Source: CAD feature listing. Evaluate the final solid. Frame: model axes, mm. A direction names the side the tool comes from. Give positions to 0.01 mm unless a question says otherwise; leave off trailing zeros. Order: outer loops, then holes, each group sorted by start corner. A loop starts at its lowest first (then second) coordinate and runs counter-clockwise, first axis right, second up.
```python
from build123d import *

# Parameters (mm, degrees)
SKETCH1_R                = 2.65
SKETCH1_R_2              = 1.65
BOSS_EXTRUDE1_DEPTH      = 6
SKETCH2_W                = 3
SKETCH2_H                = 84
BOSS_EXTRUDE2_DEPTH      = 5
BOSS_EXTRUDE2_DEPTH_BACK = 11
SKETCH3_W                = 3.872725059
SKETCH3_H                = 4
CUT_EXTRUDE2_DEPTH       = 10
CUT_EXTRUDE2_DEPTH_BACK  = 20


with BuildPart() as part:
    # Sketch1 → Boss-Extrude1 (new body)
    with BuildSketch(Plane(origin=(0, 0, 0), x_dir=(1, 0, 0), z_dir=(0, 1, 0))):
        with BuildLine():
            Line((10, 0), (0, 0))
            Line((0, 0), (0, -84))
            add(Edge.make_bspline(
                [(10, 0), (21.928320777, -51.98362607), (0, -84)],
                knots=[0, 0, 0, 0.5770461, 0.5770461, 0.5770461], degree=2))
        make_face()
        with Locations((7.5, -42.64)):
            Circle(SKETCH1_R, mode=Mode.SUBTRACT)
        with Locations((7.5, -17.64)):
            Circle(SKETCH1_R_2, mode=Mode.SUBTRACT)
    extrude(amount=BOSS_EXTRUDE1_DEPTH)

    # Sketch2 → Boss-Extrude2 (add, two sides)
    with BuildSketch(Plane(origin=(0, 6, 0), x_dir=(1, 0, 0), z_dir=(0, 1, 0))) as boss_extrude2_sk:
        with Locations((-1.5, -42)):
            Rectangle(SKETCH2_W, SKETCH2_H)
    extrude(amount=BOSS_EXTRUDE2_DEPTH)
    extrude(boss_extrude2_sk.sketch, amount=-BOSS_EXTRUDE2_DEPTH_BACK)

    # Sketch3 → Cut-Extrude2 (cut, two sides)
    with BuildSketch(Plane(origin=(0, 6, 0), x_dir=(1, 0, 0), z_dir=(0, 1, 0))) as cut_extrude2_sk:
        Polygon((23.981174241, 0), (0, 0), (0, -4), (0, -10), (23.981174241, -10), align=None)
        with Locations((-1.93636253, -2)):
            Rectangle(SKETCH3_W, SKETCH3_H)
    extrude(amount=CUT_EXTRUDE2_DEPTH, mode=Mode.SUBTRACT)
    extrude(cut_extrude2_sk.sketch, amount=-CUT_EXTRUDE2_DEPTH_BACK, mode=Mode.SUBTRACT)


solid = part.part
```
1) Section query A-A, the plane y = 5. Count the separate pieces of the cut face and the enclosed holes in it, and give its area (3 significant figures).
Report:
separate pieces: 1
enclosed holes: 2
area: 1,030 mm2
2) Reachability of faces 4 (the flat face through (6, 3, 10)), 5 (the flat face through (5, 6, 38)), 6 (the flat face through (-2, 3, 84)), 7 (the flat face through (5, 0, 38)), 8 (the flat face through (-2, 11, 43)) from +Z, -Z, +X, -X, +Y, -Y: full face, straight path, thin tool, end or side. Return the list, or none.
Report:
face 4: -Z, +X, +Y, -Y
face 5: +Z, -Z, +X, +Y
face 6: +Z, +X, -X, +Y, -Y
face 7: +Z, -Z, +X, -Y
face 8: +Z, -Z, +X, -X, +Y
3) Draft query along X for faces 1 (the flat face through (-3, 3, 45)), 2 (the cylindrical face through (7.14, 2.96, 19.25)), 3 (the flat face through (-2, -5, 43)). Return one class per face: +X half, -X half, draft (parallel to the pull), parting line (faces both ways), or undercut.
Report:
face 1: -X half
face 2: undercut
face 3: draft
4) Section query C-C, the plane y = 9.5. Return the cut outline in (x, z).
Report:
outline: (-3, 4) - (0, 4) - (0, 84) - (-3, 84) - close
5) Material intervals for L1, parallel to Z at x = 7.5, y = 4.8; L2, parallel to X at y = -1, z = 54; L3, parallel to Y at x = 6.75, z = 20, sorted ascending.
Report:
L1: z = 10 to 15.99, 19.29 to 39.99, 45.29 to 70.2
L2: x = -3 to 0
L3: y = 0 to 6
6) Pin query (flat end, axial travel): pin 1 (6 mm diameter, centred on x = 9, y = 2, fed in from -Z); pin 2 (1.5 mm diameter, centred on x = 7.5, y = 0, fed in from +Z); pin 3 (4.5 mm diameter, centred on x = 10, z = 54.5, fed in from +Y). Return the tip coordinate at first contact, or that it passes through.
Report:
pin 1: stops at z = 10
pin 2: stops at z = 71.93
pin 3: stops at y = 6
